Can you work these out from the model? Positions are in its coordinate system, mm. Give positions to 0.01 mm unless a question says otherwise; leave off trailing zeros. Order: outer loops, then holes, each group sorted by start corner. A loop starts at its lowest first (then second) coordinate and runs counter-clockwise, first axis right, second up. Notation, with made-up numbers: (87, -12) -> (91, -12) arc R11 ccw to (91, 5) -> close; hole circle Ø1 at (23.5, 69.25). An arc over 180 degrees is marked (long way). Answer as a JSON object with one key per item and string values.
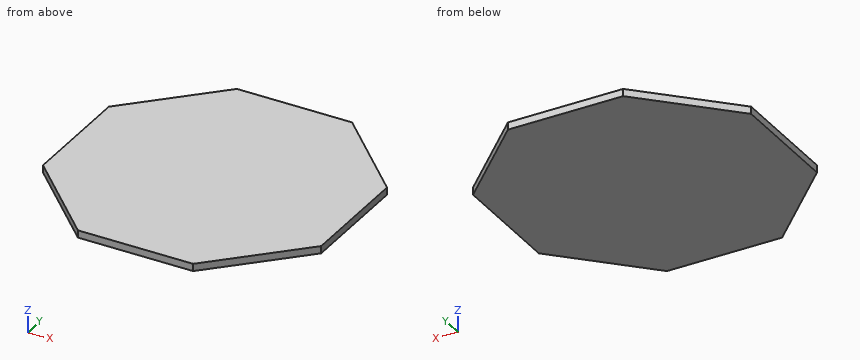
Autodesk Inventor part; units mm, degrees
ref_plane "YZ Plane" through (0, 0, 0) normal (1, 0, 0) x (0, 1, 0)
ref_plane "XZ Plane" through (0, 0, 0) normal (0, 1, 0) x (-1, 0, 0)
ref_plane "XY Plane" through (0, 0, 0) normal (0, 0, 1) x (1, 0, 0)
sketch "Sketch1" plane through (0, 0, 0) normal (0, 0, 1) x (1, 0, 0)
  circle A0 centre (0, 0) radius 57 construction
  circle A1 centre (0, 0) radius 105 construction
  line L0 (105, -105) -> (-105, -105)
  line L1 (-105, -105) -> (-105, 105)
  line L2 (-105, 105) -> (105, 105)
  line L3 (105, 105) -> (105, -105)
  line L4 (105, -105) -> (-105, 105) construction
  line L5 (-105, -105) -> (105, 105) construction
  line L6 (43.4924, 105) -> (105, 43.4924)
  line L7 (105, 43.4924) -> (105, -43.4924)
  line L8 (105, -43.4924) -> (43.4924, -105)
  line L9 (43.4924, -105) -> (-43.4924, -105)
  line L10 (-43.4924, -105) -> (-105, -43.4924)
  line L11 (-105, -43.4924) -> (-105, 43.4924)
  line L12 (-105, 43.4924) -> (-43.4924, 105)
  line L13 (-43.4924, 105) -> (43.4924, 105)
  line L14 (23.6102, 57) -> (57, 23.6102)
  line L15 (57, 23.6102) -> (57, -23.6102)
  line L16 (57, -23.6102) -> (23.6102, -57)
  line L17 (23.6102, -57) -> (-23.6102, -57)
  line L18 (-23.6102, -57) -> (-57, -23.6102)
  line L19 (-57, -23.6102) -> (-57, 23.6102)
  line L20 (-57, 23.6102) -> (-23.6102, 57)
  line L21 (-23.6102, 57) -> (23.6102, 57)
  point P0 (0, 105)
  point P1 (-105, 43.4924)
  point P2 (-43.4924, -105)
  point P3 (0, 57)
  dimension "d22" = 114
  dimension "d23" = 210
extrude "Plate1" add sketch "Sketch1" along normal blind 3 contours L14 L15 L16 L17 L18 L19 L20 L21
sketch "Sketch6" plane through (0, 0, 0) normal (0, 0, 1) x (1, 0, 0)
  line L0 (0, 0) -> (0, 85) construction
  circle A0 centre (0, 0) radius 85 construction
  line L1 (0, 0) -> (60.1041, 60.1041) construction
  circle A1 centre (60.1041, 60.1041) radius 9
  dimension "d32" = 18
  dimension "d33" = 170
  dimension "d34" = 45
cut "Cut2" [suppressed]
pattern_circular "Circular Pattern2" [suppressed]
equation "\"d23\" = Flange_D_outer"
equation "\"d32\" = Flange_d_hole_diam"
equation "\"d33\" = Flange_D1_hole_center"
equation "\"d35\" = Thickness"
equation "\"d2\" = Thickness"
equation "\"BendReliefWidth\" = Thickness"
equation "\"BendReliefDepth\" = 0.5 * Thickness"
equation "\"CornerReliefSize\" = 4 * Thickness"
equation "\"MinimumRemnant\" = 2 * Thickness"
equation "\"TransitionRadius\" = BendRadius"
equation "\"JacobiRadiusSize\" = BendRadius"
equation "\"GapSize\" = Thickness"
properties part number "210 DS-B Axis cap" material "Stainless Steel"
1. If we section it at A-A on z = 0.85: Please give me the cut outline in (x, y).
Worked answers:
{"outline": "(-57, -23.61) -> (-23.61, -57) -> (23.61, -57) -> (57, -23.61) -> (57, 23.61) -> (23.61, 57) -> (-23.61, 57) -> (-57, 23.61) -> close"}
2. If we section it at B-B on x = 42.5: Please give me the cut outline in (y, z), then the cut area to 3 significant figures.
Worked answers:
{"outline": "(-38.11, 0) -> (38.11, 0) -> (38.11, 3) -> (-38.11, 3) -> close", "area": "229 mm²"}
3. Please list where these lines run through material, in increasing order: L1, parallel to X at y = 35, z = 2.6; L2, parallel to X at y = -33.5, z = 1.7; L3, parallel to Y at x = -33, z = 1.45.
Worked answers:
{"L1": "-45.61 to 45.61", "L2": "-47.11 to 47.11", "L3": "-47.61 to 47.61"}
4. If we section it at C-C on y = 34.5: Please give me the cut outline in (x, z), then the cut area to 3 significant figures.
Worked answers:
{"outline": "(-46.11, 0) -> (46.11, 0) -> (46.11, 3) -> (-46.11, 3) -> close", "area": "277 mm²"}
5. Will this pin go through, and if not, where does the flat tip stop? pin 1 Ø1 at (x, z) = (31.5, 2.5) entering from -Y.
Worked answers:
{"pin 1": "y = -49.61"}
